Part print with two shaded views. Sizes in mm from the minimum x, y, z corner. A direction names the side the tool comes from. Give positions to 0.01 mm unless a question says otherwise; leave off trailing zeros. Loops run counter-clockwise (first coordinate to the right, second up) from the corner with the lowest first, then second, coordinate; pieces in that order, holes last. Notation, with made-up numbers: (38, 22.5) -> (70, 22.5) arc R31 cw to (70, 46.5) -> close; hole circle Ø4 at (89.25, -30). An arc over 180 degrees is marked (long way). One line per question, with ' | ' between items.
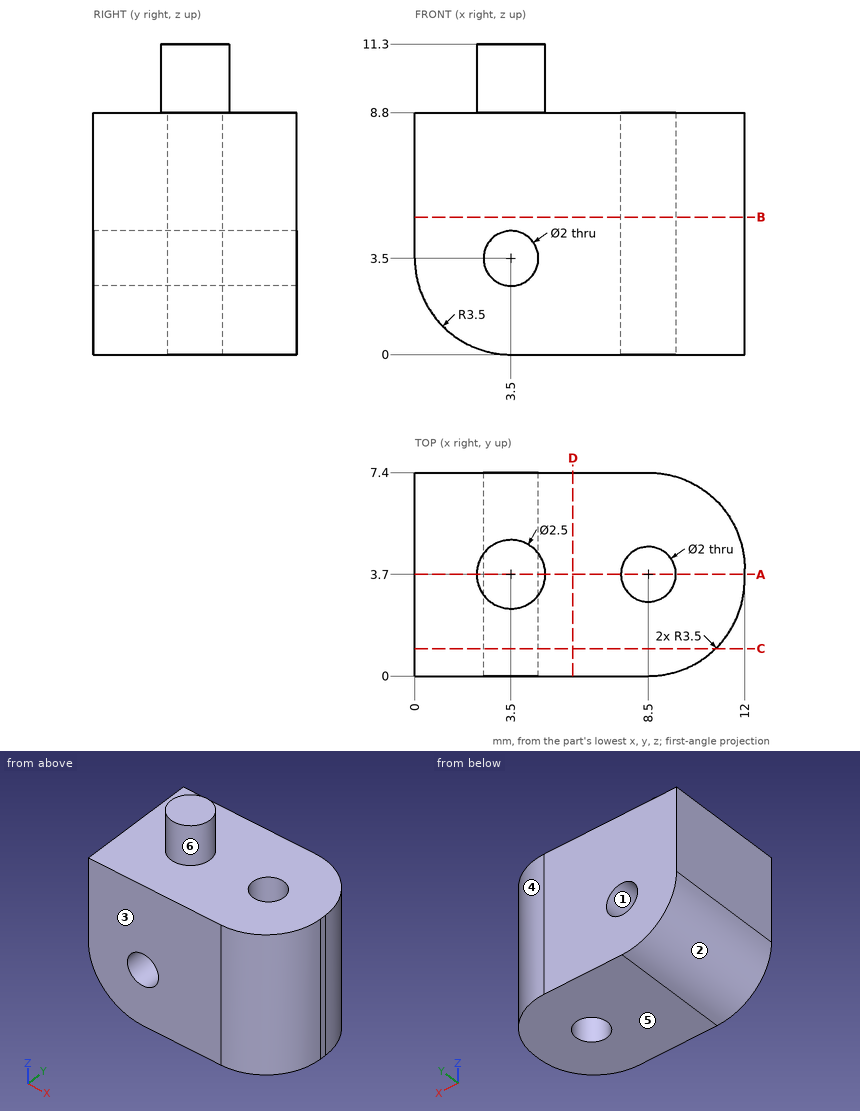
1) Pull direction X, two halves, no side cores. Call the marked faces 1, 2, 3 and 4: pulls with the +X half, pulls with the -X half, needs draft (parallel to the pull), parting line crosses it, or undercut.
Found:
face 1: undercut | face 2: pulls with the -X half | face 3: needs draft | face 4: pulls with the +X half
2) Pin check, flat tips, straight feed: P1, Ø2, axis at y = 1, z = 7.5, coming from the +X side; P2, Ø1.5, axis at x = 9.5, y = 1, coming from the +Z side. Stop position of each tip, or through.
Found:
P1: x = 11.66 | P2: z = 8.8
3) Saw through at D-D (x = 5.75). Give the cut face in (y, z), and give its area (3 significant figures).
Found:
outline: (0, 0) -> (7.4, 0) -> (7.4, 8.8) -> (0, 8.8) -> close | area: 65.1 mm2
4) Tool access for the marked faces 5 and 6: list every direction of +Z, -Z, +X, -X, +Y, -Y with a clear straight run to the whole face (end or side of a thin tool).
Found:
face 5: -Z, +X, -X, +Y, -Y | face 6: +Z
5) Drill centre lines: line 1 (Z direction, x = 3.5, y = 2); line 2 (Z direction, x = 10.5, y = 4.5); line 3 (Z direction, x = 3.5, y = 2.5). Where is each one in solid material? Low to high.
Found:
line 1: 0 to 2.5, 4.5 to 8.8 | line 2: 0 to 8.8 | line 3: 0 to 2.5, 4.5 to 11.3
6) Saw through at A-A (y = 3.7). Give the cut face in (x, z).
Found:
outline: (0, 3.5) arc R3.5 ccw to (3.5, 0) -> (7.5, 0) -> (7.5, 8.8) -> (4.75, 8.8) -> (4.75, 11.3) -> (2.25, 11.3) -> (2.25, 8.8) -> (0, 8.8) -> close; (9.5, 0) -> (12, 0) -> (12, 8.8) -> (9.5, 8.8) -> close; hole circle Ø2 at (3.5, 3.5)
7) Saw through at C-C (y = 1). Give the cut face in (x, z).
Found:
outline: (0, 3.5) arc R3.5 ccw to (3.5, 0) -> (10.95, 0) -> (10.95, 8.8) -> (0, 8.8) -> close; hole circle Ø2 at (3.5, 3.5)
8) Saw through at B-B (z = 5). Give the cut face in (x, y), and give its area (3 significant figures).
Found:
outline: (0, 0) -> (8.5, 0) arc R3.5 ccw to (12, 3.5) -> (12, 3.9) arc R3.5 ccw to (8.5, 7.4) -> (0, 7.4) -> close; hole circle Ø2 at (8.5, 3.7) | area: 80.4 mm2
